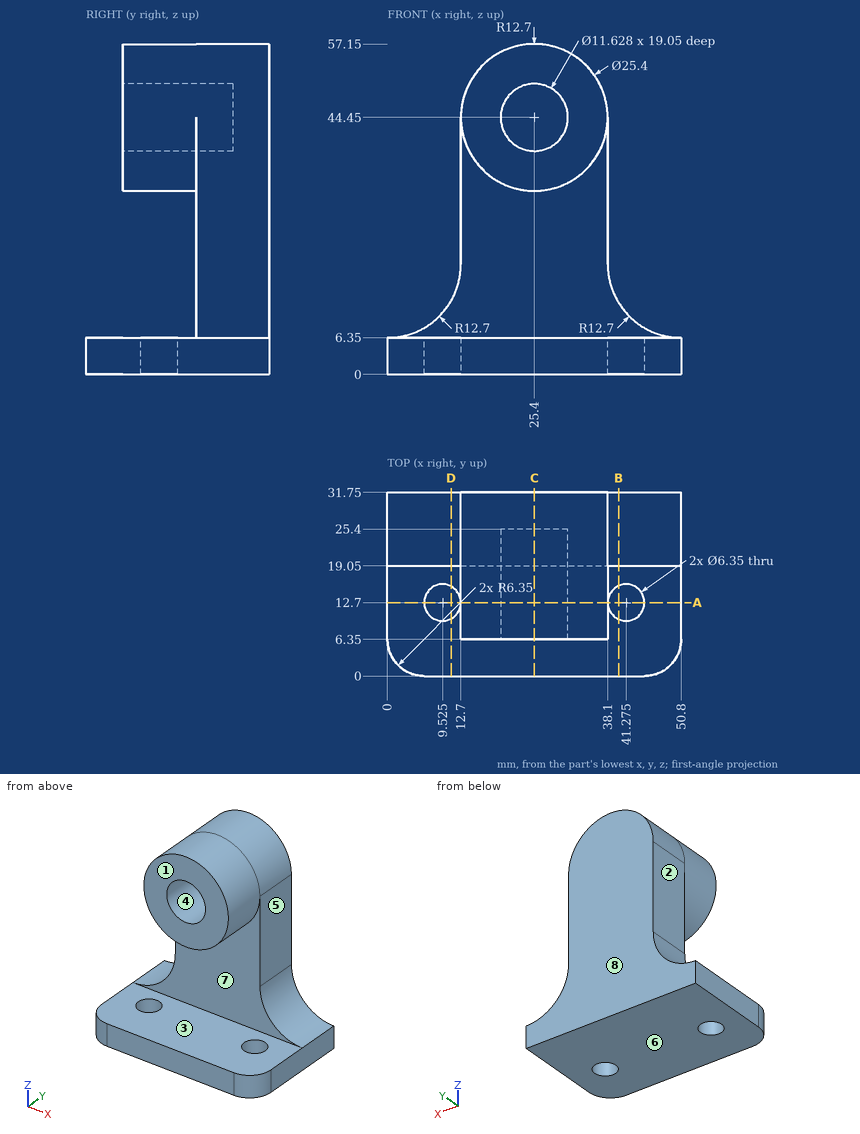
Here's the drawing with two shaded views (mm, measured from the low corner). I have some questions. A direction names the side the tool comes from. Give positions to 0.01 mm unless a question says otherwise; leave off trailing zeros. Loops run counter-clockwise (first coordinate to the right, second up) from the corner with the lowest first, then second, coordinate; pieces in that order, holes last. Notation, with made-up numbers: M -9,58 L 47,58 A24 cw 47,84 Z; hole C 74.5,30.25 d5. An arc over 180 degrees is marked long. Use one line per item in the form item = value. Start each with the question number.
Q1. I need wall thicknesses on line 1 along Z through (x, y) = (25, 17); line 2 along Z through (x, y) = (25.4, 15.75); line 3 along Y through (x, z) = (25, 10.5). Which ranges of each line are inside material? Lowest first, please.
Q2. If we section it at B-B (x = 40): Write out the boundary of the cut face in (y, z).
Q3. Thinking about a two-plate mould opening in Z: for the marked faces 6, 7 and 8, which applies, +Z half, -Z half, draft (parallel to the pull), parting line (faces both ways), or undercut?
Q4. If we section it at A-A (y = 12.7): Write out the boundary of the cut face in (x, z).
Q5. Will these pins go through, and if not, where does the flat tip stop? pin 1 Ø4 at (y, z) = (26.5, 28) entering from -X; pin 2 Ø10 at (y, z) = (24, 29) entering from +X; pin 3 Ø4 at (x, y) = (6.5, 14) entering from +Z; pin 4 Ø1 at (x, y) = (9, 28.5) entering from -Z.
Q6. If we section it at D-D (x = 11): Write out the boundary of the cut face in (y, z).
Q7. If we section it at C-C (x = 25.4): Write out the boundary of the cut face in (y, z), then the cut area to 3 significant figures.
Q8. Which directions (+Z, -Z, +X, -X, +Y, -Y) give clear straight access to the entire face, cutting with the end or side of a thin tool? Please do the marked faces 1, 2, 3, 4 and 5.
Taken from the geometry:
q1.line_1 = 0 to 6.35, 31.76 to 38.65, 50.25 to 57.14
q1.line_2 = 0 to 6.35, 31.75 to 38.64, 50.26 to 57.15
q1.line_3 = 19.05 to 31.75
q2.outline = M 0,0 L 9.79,0 L 9.79,6.35 L 0,6.35 Z; M 15.61,0 L 31.75,0 L 31.75,12.37 L 19.05,12.37 L 19.05,6.35 L 15.61,6.35 Z
q3.face_6 = -Z half
q3.face_7 = undercut
q3.face_8 = draft
q4.outline = M 0,0 L 6.35,0 L 6.35,6.35 L 0,6.35 Z; M 12.7,0 L 38.1,0 L 38.1,6.35 L 12.7,6.35 Z; C 25.4,44.45 d25.4; M 44.45,0 L 50.8,0 L 50.8,6.35 L 44.45,6.35 Z; hole C 25.4,44.45 d11.63
q5.pin_1 = 12.7
q5.pin_2 = 38.1
q5.pin_3 = 6.35
q5.pin_4 = 0
q6.outline = M 0,0 L 9.89,0 L 9.89,6.35 L 0,6.35 Z; M 15.51,0 L 31.75,0 L 31.75,12.7 L 19.05,12.7 L 19.05,6.35 L 15.51,6.35 Z
q7.outline = M 0,0 L 31.75,0 L 31.75,57.15 L 6.35,57.15 L 6.35,50.26 L 25.4,50.26 L 25.4,38.64 L 6.35,38.64 L 6.35,31.75 L 19.05,31.75 L 19.05,6.35 L 0,6.35 Z
q7.area = 948 mm^2
q8.face_1 = +Z, +X, -X, -Y
q8.face_2 = +Z, -X, +Y, -Y
q8.face_3 = +X, -X, -Y
q8.face_4 = -Y
q8.face_5 = +Z, +X, +Y, -Y
